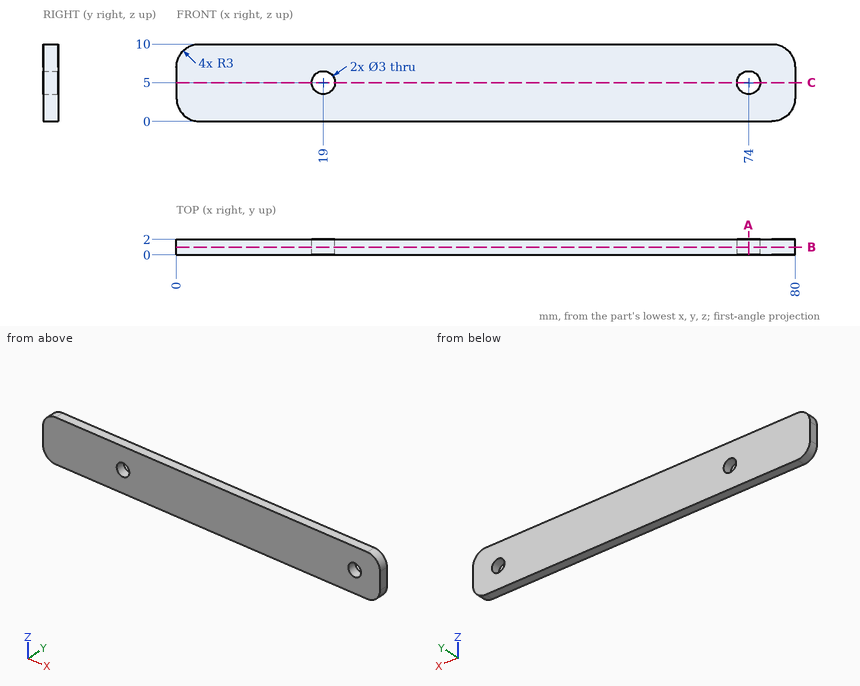
Here's the drawing with two shaded views (mm, measured from the low corner). I have some questions. Coordinates: 2 decimals unless noted, no trailing zeros. Loops run counter-clockwise (first coordinate to the right, second up) from the corner with the lowest first, then second, coordinate; pieces in that order, holes last. Notation, with made-up numbers: (-35.5, -1.75) -> (-12.5, -1.75) arc R22 ccw to (-12.5, 24.25) -> close; hole circle Ø6 at (14.5, 35.5). An arc over 180 degrees is marked (long way). Use one line per item in the form item = value. Start each with the question number.
(1) If we section it at B-B (y = 1): Please give me the cut outline in (x, z), then the cut area to 3 significant figures.
(2) Please list where these lines run through material, in increasing order: line 1 along X through (y, z) = (0.9, 5); line 2 along Z through (x, y) = (19, 0.85); line 3 along X through (y, z) = (0.3, 6).
(3) Will these pins go through, and if not, where does the flat tip stop? pin 1 (1 mm diameter, centred on x = 28.5, y = 1.5, fed in from -Z); pin 2 (2.5 mm diameter, centred on x = 19, z = 5, fed in from +Y).
(4) If we section it at C-C (z = 5): Please give me the cut outline in (x, y), then the cut area to 3 significant figures.
(5) If we section it at A-A (x = 74): Please give me the cut outline in (y, z).
Verdict:
q1.outline = (0, 3) arc R3 ccw to (3, 0) -> (77, 0) arc R3 ccw to (80, 3) -> (80, 7) arc R3 ccw to (77, 10) -> (3, 10) arc R3 ccw to (0, 7) -> close; hole circle Ø3 at (19, 5); hole circle Ø3 at (74, 5)
q1.area = 778 mm²
q2.line_1 = 0 to 17.5, 20.5 to 72.5, 75.5 to 80
q2.line_2 = 0 to 3.5, 6.5 to 10
q2.line_3 = 0 to 17.88, 20.12 to 72.88, 75.12 to 80
q3.pin_1 = 0
q3.pin_2 = through
q4.outline = (0, 0) -> (17.5, 0) -> (17.5, 2) -> (0, 2) -> close; (20.5, 0) -> (72.5, 0) -> (72.5, 2) -> (20.5, 2) -> close; (75.5, 0) -> (80, 0) -> (80, 2) -> (75.5, 2) -> close
q4.area = 148 mm²
q5.outline = (0, 0) -> (2, 0) -> (2, 3.5) -> (0, 3.5) -> close; (0, 6.5) -> (2, 6.5) -> (2, 10) -> (0, 10) -> close
